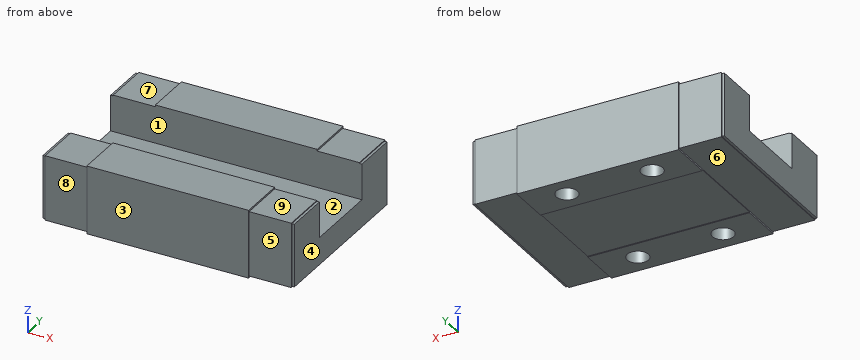
from build123d import *

# Parameters (mm, degrees)
ESQUISSE1_W                                   = 29.5
ESQUISSE1_H                                   = 20
BOSS_EXTRU_1_DEPTH                            = 4
ENL_V_MAT_EXTRU_1_DEPTH                       = 32.404617495
ENL_V_MAT_EXTRU_1_DEPTH_BACK                  = 32.404617495
ESQUISSE2_W                                   = 4.5
ESQUISSE2_H                                   = 9
ESQUISSE3_W                                   = 19
ESQUISSE3_H                                   = 10
ENL_V_MAT_EXTRU_2_DEPTH                       = 0.1
ESQUISSE4_W                                   = 5.25
ESQUISSE4_H                                   = 20
ENL_V_MAT_EXTRU_3_DEPTH                       = 0.2
ESQUISSE5_W                                   = 0.3
ESQUISSE5_H                                   = 20
ENL_V_MAT_EXTRU_4_DEPTH                       = 0.1
ESQUISSE6_W                                   = 5.25
ESQUISSE6_H                                   = 7.8
ENL_V_MAT_EXTRU_5_DEPTH                       = 0.1
ESQUISSE7_W                                   = 0.3
ESQUISSE7_H                                   = 7.8
ENL_V_MAT_EXTRU_6_DEPTH                       = 0.1
TROU_POUR_TARAUDAGE_POUR_TROU_TARAUD_M3_D     = 2.5
TROU_POUR_TARAUDAGE_POUR_TROU_TARAUD_M3_DEPTH = 4
TROU_POUR_TARAUDAGE_POUR_TROU_TARAUD_M3_TIP   = 0.751075774


with BuildPart() as part:
    # Esquisse1 → Boss.-Extru.1 (new, symmetric)
    with BuildSketch(Plane.XY):
        Rectangle(ESQUISSE1_W, ESQUISSE1_H)
    extrude(amount=BOSS_EXTRU_1_DEPTH, both=True)

    # Esquisse2 → Enlèv. mat.-Extru.1 (cut, two sides: drawn at the far end of the back side and taken through both)
    with BuildSketch(Plane(origin=(14.75, 0, 0), x_dir=(0, 0, -1), z_dir=(1, 0, 0)).offset(-ENL_V_MAT_EXTRU_1_DEPTH_BACK)):
        with Locations((-1.75, 0)):
            Rectangle(ESQUISSE2_W, ESQUISSE2_H)
    extrude(amount=ENL_V_MAT_EXTRU_1_DEPTH + ENL_V_MAT_EXTRU_1_DEPTH_BACK, mode=Mode.SUBTRACT)

    # Esquisse3 → Enlèv. mat.-Extru.2 (cut)
    with BuildSketch(Plane(origin=(0, 0, -4), x_dir=(-1, 0, 0), z_dir=(0, 0, -1))):
        Rectangle(ESQUISSE3_W, ESQUISSE3_H)
    extrude(amount=-ENL_V_MAT_EXTRU_2_DEPTH, mode=Mode.SUBTRACT)

    # Esquisse4 → Enlèv. mat.-Extru.3 (cut)
    with BuildSketch(Plane(origin=(0, 0, -4), x_dir=(-1, 0, 0), z_dir=(0, 0, -1))):
        with Locations((-12.125, 0)):
            Rectangle(ESQUISSE4_W, ESQUISSE4_H)
        with Locations((12.125, 0)):
            Rectangle(ESQUISSE4_W, ESQUISSE4_H)
    enl_v_mat_extru_3 = extrude(amount=-ENL_V_MAT_EXTRU_3_DEPTH, mode=Mode.SUBTRACT)

    # Esquisse5 → Enlèv. mat.-Extru.4 (cut)
    with BuildSketch(Plane(origin=(0, 0, -3.8), x_dir=(-1, 0, 0), z_dir=(0, 0, -1))):
        with Locations((-14.6, 0)):
            Rectangle(ESQUISSE5_W, ESQUISSE5_H)
        with Locations((14.6, 0)):
            Rectangle(ESQUISSE5_W, ESQUISSE5_H)
    enl_v_mat_extru_4 = extrude(amount=-ENL_V_MAT_EXTRU_4_DEPTH, mode=Mode.SUBTRACT)

    # Esquisse6 → Enlèv. mat.-Extru.5 (cut)
    with BuildSketch(Plane.XZ.offset(10)):
        with Locations((12.125, 0.1)):
            Rectangle(ESQUISSE6_W, ESQUISSE6_H)
        with Locations((-12.125, 0.1)):
            Rectangle(ESQUISSE6_W, ESQUISSE6_H)
    enl_v_mat_extru_5 = extrude(amount=-ENL_V_MAT_EXTRU_5_DEPTH, mode=Mode.SUBTRACT)

    # Esquisse7 → Enlèv. mat.-Extru.6 (cut)
    with BuildSketch(Plane.XZ.offset(9.9)):
        with Locations((-14.6, 0.1)):
            Rectangle(ESQUISSE7_W, ESQUISSE7_H)
        with Locations((14.6, 0.1)):
            Rectangle(ESQUISSE7_W, ESQUISSE7_H)
    enl_v_mat_extru_6 = extrude(amount=-ENL_V_MAT_EXTRU_6_DEPTH, mode=Mode.SUBTRACT)

    # Symétrie2: Enlèv. mat.-Extru.3, Enlèv. mat.-Extru.4 across plane
    add(enl_v_mat_extru_3.mirror(Plane.XY), mode=Mode.SUBTRACT)
    add(enl_v_mat_extru_4.mirror(Plane.XY), mode=Mode.SUBTRACT)

    # Symétrie2 at the second plane: Enlèv. mat.-Extru.3, Enlèv. mat.-Extru.4 across plane
    add(enl_v_mat_extru_3.mirror(Plane.ZX), mode=Mode.SUBTRACT)
    add(enl_v_mat_extru_4.mirror(Plane.ZX), mode=Mode.SUBTRACT)

    # Symétrie3: Enlèv. mat.-Extru.5, Enlèv. mat.-Extru.6 across plane
    add(enl_v_mat_extru_5.mirror(Plane.ZX), mode=Mode.SUBTRACT)
    add(enl_v_mat_extru_6.mirror(Plane.ZX), mode=Mode.SUBTRACT)

    # Trou pour taraudage pour trou taraudé M31
    with Locations(Plane(origin=(0, 0, -4), x_dir=(-1, 0, 0), z_dir=(0, 0, -1))):
        with Locations((-5, 7.5), (5, 7.5), (-5, -7.5), (5, -7.5)):
            Hole(TROU_POUR_TARAUDAGE_POUR_TROU_TARAUD_M3_D / 2, depth=TROU_POUR_TARAUDAGE_POUR_TROU_TARAUD_M3_DEPTH)
            with Locations((0, 0, -(TROU_POUR_TARAUDAGE_POUR_TROU_TARAUD_M3_DEPTH + TROU_POUR_TARAUDAGE_POUR_TROU_TARAUD_M3_TIP / 2))):  # 118° drill point
                Cone(0, TROU_POUR_TARAUDAGE_POUR_TROU_TARAUD_M3_D / 2, TROU_POUR_TARAUDAGE_POUR_TROU_TARAUD_M3_TIP, mode=Mode.SUBTRACT)


solid = part.part
Input: part model. Units: mm. Frame: model coordinates. Face numbers are marked on the shaded views. A direction names the side the tool comes from. Round coordinates to 2 decimals unless told otherwise and drop trailing zeros. Loops run counter-clockwise (first coordinate to the right, second up) from the corner with the lowest first, then second, coordinate; pieces in that order, holes last. Notation, with made-up numbers: (81.5, 76.5) -> (124.5, 76.5) arc R20 ccw to (124.5, 84.5) -> close; hole circle Ø6 at (9.25, 49.5). An arc over 180 degrees is marked (long way). Answer as a JSON object with one key per item and string values. Group by question number.
1) Section query C-C on x = 2.75. Output: boundary loops of the cut face in (y, z).
2) Section query B-B on z = -2. Output: boundary loops of the cut face in (x, y).
3) Ray query, L1, parallel to Y at x = -5, z = -2.15; L2, parallel to X at y = 7.5, z = -1.6; L3, parallel to Y at x = 1.5, z = 3. Return the intervals inside material, ascending.
4) Pin query (flat end, axial travel): pin 1 (2.5 mm diameter, centred on x = 11, y = -0.5, fed in from -Z); pin 2 (4 mm diameter, centred on x = 13, z = -1.5, fed in from -Y); pin 3 (8 mm diameter, centred on x = -9.5, y = 3.5, fed in from +Z); pin 4 (1.5 mm diameter, centred on x = -12.5, y = -7, fed in from +Z). Return the tip coordinate at first contact, or that it passes through.
5) Section query A-A on z = 1.75. Output: boundary loops of the cut face in (x, y), plus the area to 3 significant figures.
6) Section query D-D on y = -1.5. Output: boundary loops of the cut face in (x, z), plus the area to 3 significant figures.
7) Draft query along Y for the marked faces 1, 2, 3 and 4. Return one class per face: +Y half, -Y half, draft (parallel to the pull), parting line (faces both ways), or undercut.
8) Reachability of the marked faces 5, 6, 7, 8 and 9 from +Z, -Z, +X, -X, +Y, -Y: full face, straight path, thin tool, end or side. Return the list, or none.
Reply:
{
 "1": {"outline": "(-10, -4) -> (-5, -4) -> (-5, -3.9) -> (5, -3.9) -> (5, -4) -> (10, -4) -> (10, 4) -> (4.5, 4) -> (4.5, -0.5) -> (-4.5, -0.5) -> (-4.5, 4) -> (-10, 4) -> close"},
 "2": {"outline": "(-14.75, -9.8) -> (-14.45, -9.8) -> (-14.45, -9.9) -> (-9.5, -9.9) -> (-9.5, -10) -> (9.5, -10) -> (9.5, -9.9) -> (14.45, -9.9) -> (14.45, -9.8) -> (14.75, -9.8) -> (14.75, 9.8) -> (14.45, 9.8) -> (14.45, 9.9) -> (9.5, 9.9) -> (9.5, 10) -> (-9.5, 10) -> (-9.5, 9.9) -> (-14.45, 9.9) -> (-14.45, 9.8) -> (-14.75, 9.8) -> close; hole circle Ø2.5 at (-5, -7.5); hole circle Ø2.5 at (-5, 7.5); hole circle Ø2.5 at (5, -7.5); hole circle Ø2.5 at (5, 7.5)"},
 "3": {"L1": "y = -10 to -8.75, -6.25 to 6.25, 8.75 to 10", "L2": "x = -14.75 to -6.25, -3.75 to 3.75, 6.25 to 14.75", "L3": "y = -10 to -4.5, 4.5 to 10"},
 "4": {"pin 1": "stops at z = -3.8", "pin 2": "stops at y = -9.9", "pin 3": "stops at z = 4", "pin 4": "stops at z = 3.8"},
 "5": {"outline": "(-14.75, -9.8) -> (-14.45, -9.8) -> (-14.45, -9.9) -> (-9.5, -9.9) -> (-9.5, -10) -> (9.5, -10) -> (9.5, -9.9) -> (14.45, -9.9) -> (14.45, -9.8) -> (14.75, -9.8) -> (14.75, -4.5) -> (-14.75, -4.5) -> close; (-14.75, 4.5) -> (14.75, 4.5) -> (14.75, 9.8) -> (14.45, 9.8) -> (14.45, 9.9) -> (9.5, 9.9) -> (9.5, 10) -> (-9.5, 10) -> (-9.5, 9.9) -> (-14.45, 9.9) -> (-14.45, 9.8) -> (-14.75, 9.8) -> close", "area": "322 mm2"},
 "6": {"outline": "(-14.75, -3.7) -> (-14.45, -3.7) -> (-14.45, -3.8) -> (-9.5, -3.8) -> (-9.5, -3.9) -> (9.5, -3.9) -> (9.5, -3.8) -> (14.45, -3.8) -> (14.45, -3.7) -> (14.75, -3.7) -> (14.75, -0.5) -> (-14.75, -0.5) -> close", "area": "99.2 mm2"},
 "7": {"face 1": "undercut", "face 2": "undercut", "face 3": "-Y half", "face 4": "draft"},
 "8": {"face 5": "+Z, -Z, +X, -Y", "face 6": "-Z, -X, +Y, -Y", "face 7": "+Z, -X, +Y, -Y", "face 8": "+Z, -Z, -X, -Y", "face 9": "+Z, +X, +Y, -Y"}
}
